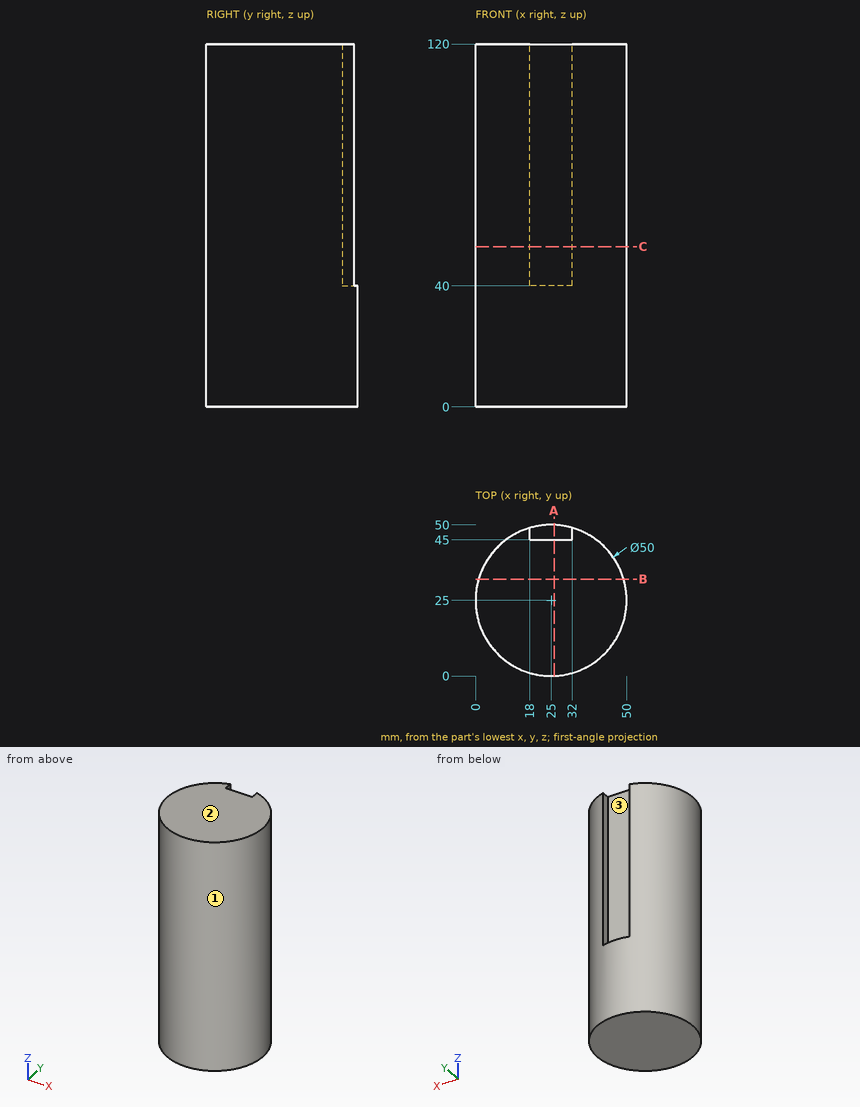
Print and shaded views of the part. All mm, measured from the part's lowest x, y and z. Coordinates: 2 decimals unless noted, no trailing zeros. Order: outer loops, then holes, each group sorted by start corner. A loop starts at its lowest first (then second) coordinate and runs counter-clockwise, first axis right, second up. Notation, with made-up numbers: (79.5, 40) -> (119.5, 40) arc R32 cw to (119.5, 77) -> close; hole circle Ø9 at (-26.75, 11). An arc over 180 degrees is marked (long way). Use one line per item in the form item = value. Start each with the question number.
1) Band-saw the part on A-A on x = 26. Give the cut face in (y, z).
2) Drill centre lines: L1, parallel to X at y = 26, z = 67.5; L2, parallel to Y at x = 29.5, z = 31. Where is each one in solid material? Low to high. Write a range as [from, to].
3) Band-saw the part on B-B on y = 32. Give the cut face in (x, z).
4) Band-saw the part on C-C on z = 53. Give the cut face in (x, y), then the cut area to 3 significant figures.
5) Pull direction X, two halves, no side cores. Call the marked faces 1, 2 and 3: +X half, -X half, draft (parallel to the pull), parting line (faces both ways), or undercut.
6) Drop flat-ended pins along their axis: pin 1 (6 mm diameter, centred on y = 38, z = 58.5, fed in from +X); pin 2 (4 mm diameter, centred on x = 25, z = 70.5, fed in from +Y); pin 3 (3 mm diameter, centred on y = 11, z = 18, fed in from +X). Give the stop position or say it passes through.
Entries:
q1.outline = (0.02, 0) -> (49.98, 0) -> (49.98, 40) -> (45, 40) -> (45, 120) -> (0.02, 120) -> close
q2.L1 = [0.02, 49.98]
q2.L2 = [0.41, 49.59]
q3.outline = (1, 0) -> (49, 0) -> (49, 120) -> (1, 120) -> close
q4.outline = (18, 45) -> (18, 49) arc R25 ccw (long way) to (32, 49) -> (32, 45) -> close
q4.area = 1,900 mm2
q5.face_1 = parting line
q5.face_2 = draft
q5.face_3 = undercut
q6.pin_1 = 47.91
q6.pin_2 = 45
q6.pin_3 = 46.65
